Design review of the part built by this model. Coordinates are the model's own, in mm. Coordinates: 2 decimals unless noted, no trailing zeros. Write each loop counter-clockwise with the first axis right and the second up, starting at its lowest first coordinate (ties: lowest second). Pieces come first, ordered by that corner, then holes. Notation, with made-up numbers: (36.5, -23.5) - (74.5, -23.5) arc R12 ccw to (74.5, -14.5) - close; hole circle Ø7 at (63, -24.5). An arc over 180 degrees is marked (long way). One line per item, written item: value.
from build123d import *

# Parameters (mm, degrees)
EXTRUDE008_DEPTH = 100


with BuildPart() as body009:
    # Sketch045 → Revolution002 (revolve)
    with BuildSketch(Plane.XZ):
        with BuildLine():
            Line((0, 0), (0, 135.563389))
            ThreePointArc((23.86226, 121.281178), (13.904936, 131.720055), (0, 135.563389))
            ThreePointArc((32.577943, 87.696618), (30.229669, 105.01041), (23.86226, 121.281178))
            ThreePointArc((22.101567, 52.101534), (30.047255, 69.102202), (32.577943, 87.696618))
            ThreePointArc((22.101567, 52.101534), (13.488015, 26.476163), (18.952965, 0))
            Line((0, 0), (18.952965, 0))
        make_face()
    revolve(axis=Axis((0, 0, 0), (0, 0, 1)))


with BuildPart() as body009_1:
    # Clone010 placement: moved
    add(body009.part.moved(Location((0, -1.1, 0))))


with BuildPart() as common007:
    # Sketch056 → Extrude008 (new body)
    with BuildSketch(Plane.XZ):
        with BuildLine():
            ThreePointArc((-17.97, 86.319116), (0, 68.349116), (17.97, 86.319116))
            ThreePointArc((17.97, 86.319116), (0, 94.009169), (-17.97, 86.319116))
        make_face()
    extrude(amount=EXTRUDE008_DEPTH)

    # Common007: intersect Body009
    add(body009_1.part, mode=Mode.INTERSECT)


solid = common007.part
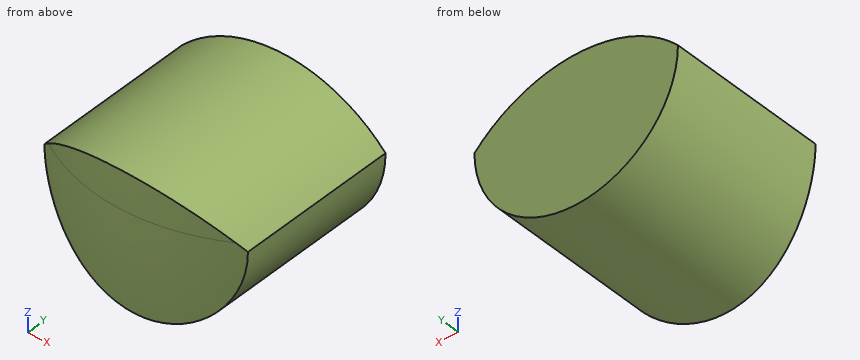
1. Consider section A-A, the plane y = -18. Write out the cut boundary in (x, z).
Answer block:
outline: (-17.97, 86.32) arc R17.97 ccw to (17.97, 86.32) arc R24.84 ccw to start
2. Insertion check: pin 1 Ø4 at (y, z) = (-24, 77.5) entering from +X; pin 2 Ø1 at (x, y) = (1, -26) entering from +Z; pin 3 Ø4 at (x, y) = (-5, -17) entering from -Z. Each pin has a flat end and moves straight along its axis. Give the tip position at first contact, or say it passes through.
Answer block:
pin 1: stops at x = 16.63
pin 2: stops at z = 94
pin 3: stops at z = 68.6
3. Wall thickness on line 1 along Z through (x, y) = (-0.5, -2.5); line 2 along Y through (x, z) = (4, 81.25); line 3 along X through (y, z) = (-17.5, 89.25): over which ranges is each line inside the solid? List them lowest first.
Answer block:
line 1: z = 68.36 to 94
line 2: y = -33.2 to 0
line 3: x = -14.62 to 14.62
